from build123d import *

# Parameters (mm, degrees)
SKETCH1_W           = 32.004
SKETCH1_H           = 98.1456
SKETCH2_R           = 31.877
BOSS_EXTRUDE1_DEPTH = 8.2296
SKETCH5_R           = 9.525
BOSS_EXTRUDE2_DEPTH = 4.572
SKETCH6_R           = 4
BOSS_EXTRUDE3_DEPTH = 31.5
SKETCH8_R           = 31.877
BOSS_EXTRUDE4_DEPTH = 8.2296
SKETCH9_R           = 15.0368
BOSS_EXTRUDE5_DEPTH = 4.7625
HOLE2_D             = 4.0386
HOLE2_DEPTH         = 13.6144
HOLE2_TIP           = 1.213317848
HOLE3_D             = 4.0386
HOLE3_DEPTH         = 13.6144
HOLE3_TIP           = 1.213317848
CHAMFER1_SIZE2      = 1.016
CHAMFER1_SIZE       = 1.015999998
FILLET1_R           = 0.254
FILLET2_R           = 1
FILLET3_R           = 1
FILLET4_R           = 1


with BuildPart() as part:
    # Sketch1 → Revolve1 (revolve)
    with BuildSketch(Plane.XZ.offset(-109.2962)):
        with Locations((51.562, -38.2524)):
            Rectangle(SKETCH1_W, SKETCH1_H)
    revolve(axis=Axis((35.56, 109.2962, 10.8204), (0, 0, -1)))

    # Sketch2 → Boss-Extrude1 (add)
    with BuildSketch(Plane.XY.offset(10.8204)):
        with Locations((35.56, 109.2962)):
            Circle(SKETCH2_R)
    extrude(amount=BOSS_EXTRUDE1_DEPTH)

    # Sketch5 → Boss-Extrude2 (add)
    with BuildSketch(Plane(origin=(0, 0, 18.542), x_dir=(-1, 0, 0), z_dir=(0, 0, -1))):
        with Locations((-35.56, 109.2962)):
            Circle(SKETCH5_R)
    extrude(amount=-BOSS_EXTRUDE2_DEPTH)

    # Sketch6 → Boss-Extrude3 (add)
    with BuildSketch(Plane.XY.offset(23.114)):
        with Locations((35.56, 109.2962)):
            Circle(SKETCH6_R)
    extrude(amount=BOSS_EXTRUDE3_DEPTH)

    # Sketch8 → Boss-Extrude4 (add)
    with BuildSketch(Plane(origin=(0, 0, -87.3252), x_dir=(-1, 0, 0), z_dir=(0, 0, -1))):
        with Locations((-35.56, 109.2962)):
            Circle(SKETCH8_R)
    extrude(amount=BOSS_EXTRUDE4_DEPTH)

    # Sketch9 → Boss-Extrude5 (add)
    with BuildSketch(Plane(origin=(0, 0, -95.5548), x_dir=(-1, 0, 0), z_dir=(0, 0, -1))):
        with Locations((-35.56, 109.2962)):
            Circle(SKETCH9_R)
    extrude(amount=BOSS_EXTRUDE5_DEPTH)

    # Hole2
    with Locations(Plane.XY.offset(19.05)):
        with Locations((60.96, 109.2962)):
            Hole(HOLE2_D / 2, depth=HOLE2_DEPTH)
            with Locations((0, 0, -(HOLE2_DEPTH + HOLE2_TIP / 2))):  # 118° drill point
                Cone(0, HOLE2_D / 2, HOLE2_TIP, mode=Mode.SUBTRACT)

    # Hole3
    with Locations(Plane.XY.offset(19.05)):
        with Locations((10.16, 109.2962)):
            Hole(HOLE3_D / 2, depth=HOLE3_DEPTH)
            with Locations((0, 0, -(HOLE3_DEPTH + HOLE3_TIP / 2))):  # 118° drill point
                Cone(0, HOLE3_D / 2, HOLE3_TIP, mode=Mode.SUBTRACT)

    # Chamfer1
    chamfer1_edges = [part.edges().sort_by_distance(p)[0] for p in [
        (45.085, 109.2962, 23.114),
    ]]
    chamfer(chamfer1_edges, length=CHAMFER1_SIZE, length2=CHAMFER1_SIZE2)

    # Fillet1
    fillet1_edges = [part.edges().sort_by_distance(p)[0] for p in [
        (31.56, 109.2962, 54.614),
    ]]
    fillet(fillet1_edges, radius=FILLET1_R)

    # Fillet2
    fillet2_edges = [part.edges().sort_by_distance(p)[0] for p in [
        (67.437, 109.2962, -95.5548),
    ]]
    fillet(fillet2_edges, radius=FILLET2_R)

    # Fillet3
    fillet3_edges = [part.edges().sort_by_distance(p)[0] for p in [
        (3.683, 109.2962, 19.05),
    ]]
    fillet(fillet3_edges, radius=FILLET3_R)

    # Fillet4
    fillet4_edges = [part.edges().sort_by_distance(p)[0] for p in [
        (50.5968, 109.2962, -100.3173),
    ]]
    fillet(fillet4_edges, radius=FILLET4_R)


solid = part.part
Geometry check sheet. Reference: the model listing, model coordinates, mm. A direction names the side the tool comes from. Coordinates: 2 decimals unless noted, no trailing zeros. Loops run counter-clockwise (first coordinate to the right, second up) from the corner with the lowest first, then second, coordinate; pieces in that order, holes last. Notation, with made-up numbers: (64, -1) - (112, -1) arc R36 cw to (112, 36) - close; hole circle Ø9 at (24, 6.25). An arc over 180 degrees is marked (long way). Use one line per item in the form item = value. Start each with the question number.
Item 1: Gauge pin test, flat ends, axial feed: pin 1 (6 mm diameter, centred on y = 103, z = 7, fed in from +X); pin 2 (4.5 mm diameter, centred on x = 60.96, y = 109.3, fed in from +Z); pin 3 (12 mm diameter, centred on x = 16, y = 103.5, fed in from -Z). Record the tip position at first contact, or that the pin passes through.
Item 2: Section check B-B, the plane z = 28.5. Enter the section's corners in (x, y), and give its area (3 significant figures).
Item 3: Tool access check on faces 1 (the face through (28.65, 78.177, 14.385)), 2 (the face through (36, 109, 54.614)), 3 (the face through (38.82, 94.617, -97.41)). Record the directions out of +Z, -Z, +X, -X, +Y, -Y that give a thin tool (end or side, any length) a straight path to the whole face; none if there is none.
Item 4: Section check C-C, the plane z = -12.5. Enter the section's corners in (x, y).
Item 5: Thickness scan on probe 1 along Z at (x, y) = (63, 102); probe 2 along Y at (x, z) = (60.96, 14.75); probe 3 along Y at (x, z) = (13, 7). Record the ranges inside material, lowest first.
Computed:
q1.pin_1 = 67.39
q1.pin_2 = 19.05
q1.pin_3 = -100.25
q2.outline = circle Ø8 at (35.56, 109.3)
q2.area = 50.3 mm2
q3.face_1 = +Z
q3.face_2 = +Z, +X, -X, +Y, -Y
q3.face_3 = -Z
q4.outline = circle Ø64.01 at (35.56, 109.3)
q5.probe_1 = -95.55 to 19.05
q5.probe_2 = 90.04 to 107.28, 111.32 to 128.56
q5.probe_3 = 86.6 to 132
